Verification items for the finished model (mm, model axes). A direction names the side the tool comes from. Coordinates: 2 decimals unless noted, no trailing zeros. Order: outer loops, then holes, each group sorted by start corner. A loop starts at its lowest first (then second) coordinate and runs counter-clockwise, first axis right, second up. Notation, with made-up numbers: (-2, 56) -> (27, 56) arc R10 cw to (27, 68) -> close; hole circle Ø8 at (81.5, -25.75). An arc over 180 degrees is marked (long way). Answer as CSV lines item,"result".
```python
from build123d import *
from build123d.topology import SkipClean

# Parameters (mm, degrees)
SKETCH1_R               = 17
SKETCH1_R_2             = 15
BOSS_EXTRUDE1_DEPTH     = 10
BOSS_EXTRUDE2_START     = 4
SKETCH5_R               = 1.5
SKETCH5_W               = 9
SKETCH5_H               = 9
BOSS_EXTRUDE2_DEPTH     = 4
CUT_EXTRUDE2_REACH      = 28.038
CUT_EXTRUDE3_DEPTH      = 27.038433133
CUT_EXTRUDE3_DEPTH_BACK = 2.4
SKETCH10_R              = 1.5
SKETCH10_R_2            = 3.45
SKETCH11_W              = 9
SKETCH11_H              = 9
CUT_EXTRUDE4_DEPTH      = 1.5


with BuildPart() as part:
    # Sketch1 → Boss-Extrude1 (new body)
    with BuildSketch(Plane(origin=(0, 0, 0), x_dir=(1, 0, 0), z_dir=(0, 1, 0))):
        with Locations(Location((0, 0, 0), (0, 0, 270))):
            Circle(SKETCH1_R)
        with Locations(Location((0, 0, 0), (0, 0, 270))):
            Circle(SKETCH1_R_2, mode=Mode.SUBTRACT)
    extrude(amount=-BOSS_EXTRUDE1_DEPTH)

    # Sketch5 → Boss-Extrude2 (add)
    with SkipClean():  # the faces are left unmerged after this step: merging them gives an invalid solid
        with BuildSketch(Plane(origin=(0, 0, 0), x_dir=(1, 0, 0), z_dir=(0, 1, 0)).offset(BOSS_EXTRUDE2_START)):
            with BuildLine():
                Line((-10.854796925, 15.981970583), (-1.723299349, 16.912428547))
                ThreePointArc((-1.723299349, 16.912428547), (0, 17), (1.723299349, 16.912428547))
                Line((1.723299349, 16.912428547), (10.854796925, 15.981970583))
                ThreePointArc((10.854796925, 15.981970583), (12.751172302, 15.179967027), (13.868467616, 13.450487203))
                Line((13.868467616, 13.450487203), (16.361128418, 4.616652129))
                ThreePointArc((16.361128418, 4.616652129), (0, -17), (-16.361128418, 4.616652129))
                Line((-16.361128418, 4.616652129), (-13.868467616, 13.450487203))
                ThreePointArc((-13.868467616, 13.450487203), (-12.751172302, 15.179967027), (-10.854796925, 15.981970583))
            make_face()
            with Locations(Location((-10.5, 0, 0), (0, 0, 270))):
                Circle(SKETCH5_R, mode=Mode.SUBTRACT)
            with Locations(Location((10.5, 0, 0), (0, 0, 270))):
                Circle(SKETCH5_R, mode=Mode.SUBTRACT)
            with Locations(Location((-10.5, 12.5, 0), (0, 0, 64.453929983))):
                Circle(SKETCH5_R, mode=Mode.SUBTRACT)
            with Locations(Location((10.5, 12.5, 0), (0, 0, 115.546070017))):
                Circle(SKETCH5_R, mode=Mode.SUBTRACT)
            Rectangle(SKETCH5_W, SKETCH5_H, mode=Mode.SUBTRACT)
        extrude(amount=-BOSS_EXTRUDE2_DEPTH)

    # Sketch9 → Cut-Extrude2 (cut, up to next)
    with BuildSketch(Plane.XZ, mode=Mode.PRIVATE) as cut_extrude2_sk1:
        with BuildLine():
            Line((7.5, 12.990381057), (8.5, 14.722431864))
            ThreePointArc((8.5, 14.722431864), (0, 17), (-8.5, 14.722431864))
            Line((-8.5, 14.722431864), (-7.5, 12.990381057))
            ThreePointArc((-7.5, 12.990381057), (0, 15), (7.5, 12.990381057))
        make_face()
    cut_extrude2_tool1 = extrude(cut_extrude2_sk1.sketch, amount=CUT_EXTRUDE2_REACH, mode=Mode.PRIVATE) & part.part
    # Sketch9 → Cut-Extrude2 (cut, up to next)
    with BuildSketch(Plane.XZ, mode=Mode.PRIVATE) as cut_extrude2_sk2:
        with BuildLine():
            Line((7.5, -12.990381057), (8.5, -14.722431864))
            ThreePointArc((8.5, -14.722431864), (14.722431864, -8.5), (17, 0))
            Line((17, 0), (15, 0))
            ThreePointArc((15, 0), (12.990381057, -7.5), (7.5, -12.990381057))
        make_face()
    cut_extrude2_tool2 = extrude(cut_extrude2_sk2.sketch, amount=CUT_EXTRUDE2_REACH, mode=Mode.PRIVATE) & part.part
    # Sketch9 → Cut-Extrude2 (cut, up to next)
    with BuildSketch(Plane.XZ, mode=Mode.PRIVATE) as cut_extrude2_sk3:
        with BuildLine():
            Line((-7.5, -12.990381057), (-8.5, -14.722431864))
            ThreePointArc((-8.5, -14.722431864), (-14.722431864, -8.5), (-17, 0))
            Line((-17, 0), (-15, 0))
            ThreePointArc((-15, 0), (-12.990381057, -7.5), (-7.5, -12.990381057))
        make_face()
    cut_extrude2_tool3 = extrude(cut_extrude2_sk3.sketch, amount=CUT_EXTRUDE2_REACH, mode=Mode.PRIVATE) & part.part
    add(cut_extrude2_tool1.solids().sort_by_distance((0, 0, 15.298769))[0], mode=Mode.SUBTRACT)
    add(cut_extrude2_tool2.solids().sort_by_distance((13.249123, 0, -7.649384))[0], mode=Mode.SUBTRACT)
    add(cut_extrude2_tool3.solids().sort_by_distance((-13.249123, 0, -7.649384))[0], mode=Mode.SUBTRACT)

    # Sketch10 → Cut-Extrude3 (cut, two sides: drawn at the far end of the back side and taken through both)
    # profile 1 of 4: a face of its own
    with SkipClean():  # the faces are left unmerged after this step: merging them gives an invalid solid
        with BuildSketch(Plane.XZ.offset(-CUT_EXTRUDE3_DEPTH_BACK)):
            with BuildLine():
                Line((-16.361128418, -4.616652129), (-13.868467616, -13.450487203))
                ThreePointArc((-13.868467616, -13.450487203), (-12.751172302, -15.179967027), (-10.854796925, -15.981970583))
                Line((-10.854796925, -15.981970583), (-1.723299349, -16.912428547))
                ThreePointArc((-1.723299349, -16.912428547), (-4.822527429, -16.301632716), (-7.755248385, -15.127991357))
                ThreePointArc((-7.755248385, -15.127991357), (-8.055870072, -9.590321514), (-13.562312591, -10.250057424))
                ThreePointArc((-13.562312591, -10.250057424), (-15.224549066, -7.563934541), (-16.361128418, -4.616652129))
            make_face()
            with Locations(Location((-10.5, -12.5, 0), (0, 0, 270))):
                Circle(SKETCH10_R, mode=Mode.SUBTRACT)
        # profile 2 of 4: a face of its own
        with BuildSketch(Plane.XZ.offset(-CUT_EXTRUDE3_DEPTH_BACK)):
            with BuildLine():
                ThreePointArc((7.755248385, -15.127991357), (4.822527429, -16.301632716), (1.723299349, -16.912428547))
                Line((1.723299349, -16.912428547), (10.854796925, -15.981970583))
                ThreePointArc((10.854796925, -15.981970583), (12.751172302, -15.179967027), (13.868467616, -13.450487203))
                Line((13.868467616, -13.450487203), (16.361128418, -4.616652129))
                ThreePointArc((16.361128418, -4.616652129), (15.224549066, -7.563934541), (13.562312591, -10.250057424))
                ThreePointArc((13.562312591, -10.250057424), (8.055870072, -9.590321514), (7.755248385, -15.127991357))
            make_face()
            with Locations(Location((10.5, -12.5, 0), (0, 0, 270))):
                Circle(SKETCH10_R, mode=Mode.SUBTRACT)
        # profile 3 of 4: a face of its own
        with BuildSketch(Plane.XZ.offset(-CUT_EXTRUDE3_DEPTH_BACK)):
            with Locations(Location((-10.5, 0, 0), (0, 0, 90))):
                Circle(SKETCH10_R_2)
            with Locations(Location((-10.5, 0, 0), (0, 0, 270))):
                Circle(SKETCH10_R, mode=Mode.SUBTRACT)
        # profile 4 of 4: a face of its own
        with BuildSketch(Plane.XZ.offset(-CUT_EXTRUDE3_DEPTH_BACK)):
            with Locations(Location((10.5, 0, 0), (0, 0, 90))):
                Circle(SKETCH10_R_2)
            with Locations(Location((10.5, 0, 0), (0, 0, 270))):
                Circle(SKETCH10_R, mode=Mode.SUBTRACT)
        extrude(amount=CUT_EXTRUDE3_DEPTH + CUT_EXTRUDE3_DEPTH_BACK, mode=Mode.SUBTRACT)

    # Sketch11 → Cut-Extrude4 (cut)
    with SkipClean():  # the faces are left unmerged after this step: merging them gives an invalid solid
        with BuildSketch(Plane(origin=(0, 4, 0), x_dir=(1, 0, 0), z_dir=(0, 1, 0))):
            with Locations((0, 9)):
                Rectangle(SKETCH11_W, SKETCH11_H)
        extrude(amount=-CUT_EXTRUDE4_DEPTH, mode=Mode.SUBTRACT)


solid = part.part
```
Item 1: Thickness scan on line 1 (X direction, y = 1.1, z = 0); line 2 (X direction, y = 3.55, z = 0); line 3 (X direction, y = -3.5, z = 0.5). Record the ranges inside material, lowest first.
Answer list:
line 1,"-17 to -13.95, -7.05 to -4.5, 4.5 to 7.05, 13.95 to 17"
line 2,"-17 to -12, -9 to -4.5, 4.5 to 9, 12 to 17"
line 3,"-16.99 to -14.99, 14.99 to 16.99"
Item 2: Release check for a two-part mould opening along Z. For faces 5 (the flat face through (-15.132, 3.211, -8.972)), 6 (the flat face through (7.99, -4.93, 13.84)), 7 (the flat face through (0, 4, 7)), 8 (the flat face through (4.5, 2, -2)) record: +Z half, -Z half, draft (parallel to the pull), parting line (faces both ways), or undercut.
Answer list:
face 5,"-Z half"
face 6,"+Z half"
face 7,"draft"
face 8,"undercut"
Item 3: Depth check by flat-ended pin: pin 1 Ø2 at (x, y) = (-15.5, -5.5) entering from -Z; pin 2 Ø3.5 at (x, z) = (-11.5, -0.5) entering from -Y; pin 3 Ø3 at (x, y) = (-10, 0) entering from +Z. Enter the tip coordinate at first touch or a pass-through.
Answer list:
pin 1,"z = 0"
pin 2,"y = 2.4"
pin 3,"z = 14.72"
Item 4: Section check C-C, the plane y = -1.75. Record the boundary of the cut face in (x, z), plus the area to 3 significant figures.
Answer list:
outline,"(-17, 0) -> (-15, 0) arc R15 cw to (-7.5, 12.99) -> (-8.5, 14.72) arc R17 ccw to start; (-7.76, -15.13) arc R17 ccw to (7.76, -15.13) arc R3.8 cw to (6.8, -13.37) arc R15 cw to (-6.8, -13.37) arc R3.8 cw to start; (7.5, 12.99) arc R15 cw to (15, 0) -> (17, 0) arc R17 ccw to (8.5, 14.72) -> close"
area,"96.9 mm2"
Item 5: Section check A-A, the plane x = 0. Record the boundary of the cut face in (y, z), plus the area to 4 significant figures.
Answer list:
outline,"(-10, -17) -> (4, -17) -> (4, -13.5) -> (2.5, -13.5) -> (2.5, -4.5) -> (0, -4.5) -> (0, -15) -> (-10, -15) -> close; (0, 4.5) -> (4, 4.5) -> (4, 17) -> (0, 17) -> close"
area,"106.5 mm2"
Item 6: Tool access check on faces 1 (the flat face through (11.2, 2.4, 1.5)), 2 (the flat face through (0, 2.5, -9)), 3 (the flat face through (0, 1, -4.5)), 4 (the flat face through (-16, -5, 0)). Record the directions out of +Z, -Z, +X, -X, +Y, -Y that give a thin tool (end or side, any length) a straight path to the whole face; none if there is none.
Answer list:
face 1,"-Y"
face 2,"+Y"
face 3,"+Y, -Y"
face 4,"-Z, +X, -X, -Y"
Item 7: Section check D-D, the plane z = -12.5. Record the boundary of the cut face in (x, y), plus the area to 3 significant figures.
Answer list:
outline,"(-14.14, 2.4) -> (-12, 2.4) -> (-12, 4) -> (-14.14, 4) -> close; (-9, 2.4) -> (-6.7, 2.4) -> (-6.7, 0) -> (6.7, 0) -> (6.7, 2.4) -> (9, 2.4) -> (9, 4) -> (4.5, 4) -> (4.5, 2.5) -> (-4.5, 2.5) -> (-4.5, 4) -> (-9, 4) -> close; (12, 2.4) -> (14.14, 2.4) -> (14.14, 4) -> (12, 4) -> close"
area,"54.3 mm2"
Item 8: Section check B-B, the plane y = 1. Record the boundary of the cut face in (x, z), plus the area to 3 significant figures.
Answer list:
outline,"(-13.56, -10.25) arc R3.8 cw (long way) to (-7.76, -15.13) arc R17 ccw to (7.76, -15.13) arc R3.8 cw (long way) to (13.56, -10.25) arc R17 ccw (long way) to start; hole circle Ø6.9 at (-10.5, 0); hole (-4.5, -4.5) -> (4.5, -4.5) -> (4.5, 4.5) -> (-4.5, 4.5) -> close; hole circle Ø6.9 at (10.5, 0)"
area,"699 mm2"
